Part model, mm, in its own coordinate system. A direction names the side the tool comes from. Give positions to 0.01 mm unless a question says otherwise; leave off trailing zeros. Order: outer loops, then holes, each group sorted by start corner. A loop starts at its lowest first (then second) coordinate and runs counter-clockwise, first axis right, second up.
Autodesk Inventor part; units mm, degrees
ref_plane "YZ Plane" through (0, 0, 0) normal (1, 0, 0) x (0, 1, 0)
ref_plane "XZ Plane" through (0, 0, 0) normal (0, 1, 0) x (-1, 0, 0)
ref_plane "XY Plane" through (0, 0, 0) normal (0, 0, 1) x (1, 0, 0)
sketch "Sketch1" plane through (0, 0, 0) normal (0, 1, 0) x (-1, 0, 0)
  line L0 (-50.8, 50.8) -> (50.8, 50.8)
  line L1 (50.8, 50.8) -> (50.8, -50.8)
  line L2 (50.8, -50.8) -> (-50.8, -50.8)
  line L3 (-50.8, -50.8) -> (-50.8, 50.8)
  line L4 (-50.8, 50.8) -> (50.8, -50.8) construction
  line L5 (50.8, 50.8) -> (-50.8, -50.8) construction
  line L6 (76.2, -76.2) -> (76.2, 76.2)
  line L7 (76.2, 76.2) -> (-76.2, 76.2)
  line L8 (-76.2, 76.2) -> (-76.2, -76.2)
  line L9 (-76.2, -76.2) -> (76.2, -76.2)
  point P0 (0, 0)
  dimension "d0" = 101.6
  dimension "d1" = 101.6
  dimension "d2" = 25.4
extrude "Extrusion1" add sketch "Sketch1" along normal blind 152.4
chamfer "Chamfer1" distance 25.4 distance2 152.4 1 edges at (0, 152.4, 76.2) measured on face at (-16.9333, 152.4, -67.7333)
chamfer "Chamfer2" distance 25.4 distance2 152.4 1 edges at (76.2, 152.4, -12.6998) measured on face at (-16.9333, 152.4, -67.7333)
chamfer "Chamfer3" distance 25.4 distance2 152.4 1 edges at (-12.6998, 152.4, -76.2) measured on face at (-25.3998, 152.4, -67.7333)
chamfer "Chamfer4" distance 25.4 distance2 152.4 1 edges at (-76.2, 152.4, 0) measured on face at (-67.7333, 152.4, -16.9333)
properties part number "PostBase" material "Iron, Cast"
Item 1: Band-saw the part on D-D on y = 119. List the corners of the cut face in (x, z), plus the area to 3 significant figures.
Item 2: Which spindle directions (+Z, -Z, +X, -X, +Y, -Y) get a long thin tool onto all of the face, cutting with end or side? Do faces 1 (the face through (1, 75, 50.8)), 2 (the face through (1.07, 75.13, -63.68)). Say none if no direction does.
Item 3: Band-saw the part on C-C on y = 13.5. List the corners of the cut face in (x, z), plus the area to 3 significant figures.
Item 4: Drop flat-ended pins along their axis: P1, Ø12, axis at y = 54.5, z = -25, coming from the +X side; P2, Ø6, axis at x = -2.5, z = -53.5, coming from the -Y side; P3, Ø3, axis at y = 51, z = -42.5, coming from the -X side; P4, Ø4, axis at x = 40.5, y = 101, coming from the +Z side. Give the stop position or say it passes through.
Item 5: Drill centre lines: probe 1 along Z at (x, y) = (48, 35); probe 2 along Z at (x, y) = (-30, 108.5); probe 3 along X at (y, z) = (143, 38.5). Where is each one in solid material? Low to high.
Item 6: Pull direction Z, two halves, no side cores. Call faces 3 (the face through (-50.8, 75, 1)), 4 (the face through (52, 0, 1)), 5 (the face through (-1.07, 75.13, 63.68)): released by +Z, released by -Z, zero draft, split by the parting line, or undercut.
Working result:
1. outline: (-56.37, -56.37) - (56.37, -56.37) - (56.37, 56.37) - (-56.37, 56.37) - close; hole (-50.8, -50.8) - (50.8, -50.8) - (50.8, 50.8) - (-50.8, 50.8) - close
1. area: 2,390 mm2
2. face 1: +Y, -Y
2. face 2: -Z, +X, -X, +Y
3. outline: (-73.95, -73.95) - (73.95, -73.95) - (73.95, 73.95) - (-73.95, 73.95) - close; hole (-50.8, -50.8) - (50.8, -50.8) - (50.8, 50.8) - (-50.8, 50.8) - close
3. area: 11,600 mm2
4. P1: stops at x = 68.12
4. P2: stops at y = 0
4. P3: stops at x = -67.95
4. P4: stops at z = 59.7
5. probe 1: z = -70.37 to -50.8, 50.8 to 70.37
5. probe 2: z = -58.12 to -50.8, 50.8 to 58.12
5. probe 3: x = -52.37 to -50.8, 50.8 to 52.37
6. face 3: undercut
6. face 4: zero draft
6. face 5: released by +Z
